Read the model definition and answer for the solid it produces. Units are mm, in the model's axes. A direction names the side the tool comes from. Coordinates: 2 decimals unless noted, no trailing zeros. Order: outer loops, then holes, each group sorted by start corner. A loop starts at its lowest first (then second) coordinate and runs counter-clockwise, first axis right, second up. Notation, with made-up numbers: (32, 30) - (91, 30) arc R37 ccw to (91, 67) - close; hole circle Ø8 at (72, 89.5). An arc over 180 degrees is marked (long way). Use one line per item in the form item = value.
```python
from build123d import *

# Parameters (mm, degrees)
BOSS_EXTRUDE1_DEPTH = 12
SKETCH2_W           = 20
SKETCH2_H           = 20
BOSS_EXTRUDE2_DEPTH = 60
SKETCH3_W           = 38.284232122
SKETCH3_H           = 32.888854422
BOSS_EXTRUDE3_DEPTH = 2


with BuildPart() as part:
    # Sketch1 → Boss-Extrude1 (new body)
    with BuildSketch(Plane(origin=(0, 0, 0), x_dir=(1, 0, 0), z_dir=(0, 1, 0))):
        Polygon((0, 5.773502692), (-5, 2.886751346), (-5, -2.886751346), (0, -5.773502692), (5, -2.886751346), (5, 2.886751346), align=None)
    extrude(amount=BOSS_EXTRUDE1_DEPTH)

    # Sketch2 → Boss-Extrude2 (add)
    with BuildSketch(Plane(origin=(0, 12, 0), x_dir=(1, 0, 0), z_dir=(0, 1, 0))):
        Rectangle(SKETCH2_W, SKETCH2_H)
    extrude(amount=BOSS_EXTRUDE2_DEPTH)

    # Sketch3 → Boss-Extrude3 (add)
    with BuildSketch(Plane(origin=(0, 72, 0), x_dir=(1, 0, 0), z_dir=(0, 1, 0))):
        Rectangle(SKETCH3_W, SKETCH3_H)
    extrude(amount=BOSS_EXTRUDE3_DEPTH)


solid = part.part
```
(1) Given pin 1 Ø4 at (x, y) = (9, 53.5) entering from +Z; pin 2 Ø1.5 at (x, y) = (7.5, 47.5) entering from -Z; pin 3 Ø12 at (x, z) = (-14.5, -5) entering from -Y, each flat-ended and moving along its own axis, determine where each tip first touches the part or whether it passes through.
Answer list:
pin_1 = 10
pin_2 = -10
pin_3 = 12
(2) Section C-C, the plane y = 47 is taken. Write down the section's boundary in (x, z).
Answer list:
outline = (-10, -10) - (10, -10) - (10, 10) - (-10, 10) - close
(3) Section D-D, the plane x = 2.5 is taken. Write down the section's boundary in (y, z), then the cut area to 3 significant figures.
Answer list:
outline = (0, -4.33) - (12, -4.33) - (12, -10) - (72, -10) - (72, -16.44) - (74, -16.44) - (74, 16.44) - (72, 16.44) - (72, 10) - (12, 10) - (12, 4.33) - (0, 4.33) - close
area = 1,370 mm2
(4) Straight lines are drawn through the part: L1, parallel to Y at x = -2, z = 6; L2, parallel to Y at x = -16.5, z = -13; L3, parallel to Z at x = -2.5, y = 33. For each, find the intervals that lie inside material, in ascending order.
Answer list:
L1 = 12 to 74
L2 = 72 to 74
L3 = -10 to 10
(5) Section B-B, the plane x = 6.5 is taken. Write down the section's boundary in (y, z).
Answer list:
outline = (12, -10) - (72, -10) - (72, -16.44) - (74, -16.44) - (74, 16.44) - (72, 16.44) - (72, 10) - (12, 10) - close
(6) Section A-A, the plane z = -1.5 is taken. Write down the section's boundary in (x, y).
Answer list:
outline = (-19.14, 72) - (-10, 72) - (-10, 12) - (-5, 12) - (-5, 0) - (5, 0) - (5, 12) - (10, 12) - (10, 72) - (19.14, 72) - (19.14, 74) - (-19.14, 74) - close
(7) Which of the six approach directions +Z, -Z, +X, -X, +Y, -Y give full straight-line access (tool end or side, diameter ignored) to faces 1 (the flat face through (5, 6, 0)), 2 (the flat face through (0, 42, 10)), 3 (the flat face through (-10, 42, 0)), 4 (the flat face through (-2.535, 5.916, 4.31)), 5 (the flat face through (0, 42, -10))?
Answer list:
face_1 = +Z, -Z, +X, -Y
face_2 = +Z, +X, -X, -Y
face_3 = +Z, -Z, -X, -Y
face_4 = +Z, -X, -Y
face_5 = -Z, +X, -X, -Y
